The model under review builds one solid part; all positions refer to its coordinate system, in mm. Face numbers are marked on the shaded views. A direction names the side the tool comes from. Round coordinates to 2 decimals unless told otherwise and drop trailing zeros. Order: outer loops, then holes, each group sorted by start corner. A loop starts at its lowest first (then second) coordinate and runs counter-clockwise, first axis right, second up.
1) To check wall thickness, follow L1, parallel to Z at x = 20, y = -2.75; L2, parallel to X at y = 8, z = 30; L3, parallel to Z at x = 90, y = -4. State the ranges of each line that lie inside material, in increasing order.
2) Consider section D-D (y = -3.5). Give the boundary of the cut face in (x, z), then the cut area to 3 significant figures.
3) Consider section C-C (z = 28.5). Give the boundary of the cut face in (x, y).
4) Clearance check with flat-ended pins moving along their axes: P1, Ø2, axis at x = 73, y = 5, coming from the -Z side; P2, Ø5, axis at y = 2, z = -30.5, coming from the +X side; P3, Ø5, axis at x = 58, y = -2, coming from the +Z side; P4, Ø6, axis at x = 21.5, z = 30.5, coming from the +Y side. State where each tip first meets the part, or that it passes through.
5) Machinability: for the marked faces 1, 2, 3 and 4, which of the approach directions +Z, -Z, +X, -X, +Y, -Y give a long, thin tool a straight path to every point of the face, cutting with its end or side? Answer none if there is none.
6) Consider section B-B (z = -10). Give the boundary of the cut face in (x, y), then the cut area to 3 significant figures.
7) Mouldability with a two-part tool opening along X and no side actions: class the marked faces 5, 6, 7 and 8 as pulls with the +X half, pulls with the -X half, needs draft (parallel to the pull), parting line crosses it, or undercut.
8) Consider section A-A (y = 4.5). Give the boundary of the cut face in (x, z), then the cut area to 3 significant figures.
from build123d import *

# Parameters (mm, degrees)
BOSS_EXTRUDE2_DEPTH = 10
SKETCH3_R           = 10
CUT_EXTRUDE1_DEPTH  = 10
SKETCH4_R           = 5
CUT_EXTRUDE2_DEPTH  = 21


with BuildPart() as part:
    # Sketch2 → Boss-Extrude2 (new body, symmetric)
    with BuildSketch(Plane(origin=(0, 0, 0), x_dir=(1, 0, 0), z_dir=(0, 1, 0))):
        with BuildLine():
            Line((5, -30), (5, -15))
            Line((5, -15), (0, -15))
            ThreePointArc((0, -15), (-10.606601718, -10.606601718), (-15, 0))
            Line((-15, 0), (-15, 20))
            ThreePointArc((-15, 20), (-10.606601718, 30.606601718), (0, 35))
            Line((0, 35), (5, 35))
            Line((5, 35), (5, 50))
            ThreePointArc((5, 50), (20, 65), (35, 50))
            Line((35, 50), (35, 25))
            Line((35, 25), (90, 25))
            ThreePointArc((90, 25), (105, 10), (90, -5))
            Line((90, -5), (35, -5))
            Line((35, -5), (35, -30))
            ThreePointArc((35, -30), (20, -45), (5, -30))
        make_face()
        with BuildLine():
            Line((7.5, 20), (7.5, 0))
            ThreePointArc((7.5, 0), (0, -7.5), (-7.5, 0))
            Line((-7.5, 0), (-7.5, 20))
            ThreePointArc((-7.5, 20), (0, 27.5), (7.5, 20))
        make_face(mode=Mode.SUBTRACT)
    extrude(amount=BOSS_EXTRUDE2_DEPTH, both=True)

    # Sketch3 → Cut-Extrude1 (cut)
    with BuildSketch(Plane(origin=(0, 10, 0), x_dir=(1, 0, 0), z_dir=(0, 1, 0))):
        with Locations((90, 10)):
            Circle(SKETCH3_R)
        with Locations((20, 50)):
            Circle(SKETCH3_R)
        with Locations((20, -30)):
            Circle(SKETCH3_R)
    extrude(amount=-CUT_EXTRUDE1_DEPTH, mode=Mode.SUBTRACT)

    # Sketch4 → Cut-Extrude2 (cut, through all)
    with BuildSketch(Plane(origin=(0, 10, 0), x_dir=(1, 0, 0), z_dir=(0, 1, 0))):
        with Locations((20, 50)):
            Circle(SKETCH4_R)
        with Locations((20, -30)):
            Circle(SKETCH4_R)
        with Locations((90, 10)):
            Circle(SKETCH4_R)
    extrude(amount=-CUT_EXTRUDE2_DEPTH, mode=Mode.SUBTRACT)


solid = part.part
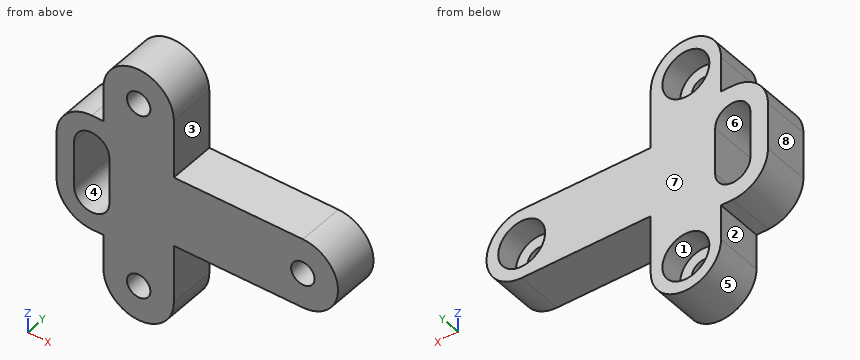
Answer below:
1. L1: z = -65 to -55, -45 to 25, 35 to 45
1. L2: x = 5 to 10, 30 to 35
1. L3: z = -25 to -15, -5 to 5
2. outline: (-15, -20) arc R15 ccw to (0, -35) - (5, -35) - (5, -50) arc R15 ccw to (35, -50) - (35, -25) - (90, -25) arc R15 ccw to (90, 5) - (35, 5) - (35, 30) arc R15 ccw to (5, 30) - (5, 15) - (0, 15) arc R15 ccw to (-15, 0) - close; hole (-7.5, -20) arc R7.5 ccw to (7.5, -20) - (7.5, 0) arc R7.5 ccw to (-7.5, 0) - close; hole circle Ø10 at (20, -50); hole circle Ø10 at (20, 30); hole circle Ø10 at (90, -10)
2. area: 5,300 mm2
3. outline: (5, -10) - (15.23, -10) - (15.23, 0) - (10.11, 0) - (10.11, 10) - (5, 10) - close; (24.77, -10) - (35, -10) - (35, 10) - (29.89, 10) - (29.89, 0) - (24.77, 0) - close
4. P1: stops at z = -25
4. P2: stops at x = 35
4. P3: stops at z = 5
4. P4: passes through
5. face 1: +Y
5. face 2: -Z, -X, +Y, -Y
5. face 3: +Z, +X, +Y, -Y
5. face 4: +Y, -Y
6. outline: (-15, -10) - (-7.5, -10) - (-7.5, 10) - (-15, 10) - close; (7.5, -10) - (85, -10) - (85, 0) - (80, 0) - (80, 10) - (7.5, 10) - close; (95, -10) - (105, -10) - (105, 10) - (100, 10) - (100, 0) - (95, 0) - close
6. area: 1,800 mm2
7. face 5: parting line crosses it
7. face 6: undercut
7. face 7: needs draft
7. face 8: pulls with the -X half
8. outline: (-15, -20) arc R15 ccw to (0, -35) - (5, -35) - (5, -50) arc R15 ccw to (35, -50) - (35, -25) - (90, -25) arc R15 ccw to (90, 5) - (35, 5) - (35, 30) arc R15 ccw to (5, 30) - (5, 15) - (0, 15) arc R15 ccw to (-15, 0) - close; hole (-7.5, -20) arc R7.5 ccw to (7.5, -20) - (7.5, 0) arc R7.5 ccw to (-7.5, 0) - close; hole circle Ø20 at (20, -50); hole circle Ø20 at (20, 30); hole circle Ø20 at (90, -10)
8. area: 4,590 mm2
